The listing builds one solid part. Answer for the finished solid, in the listing's coordinates (mm). Face numbers are marked on the shaded views. A direction names the side the tool comes from. Coordinates: 2 decimals unless noted, no trailing zeros. Order: outer loops, then holes, each group sorted by start corner. A loop starts at its lowest first (then second) coordinate and runs counter-clockwise, first axis right, second up.
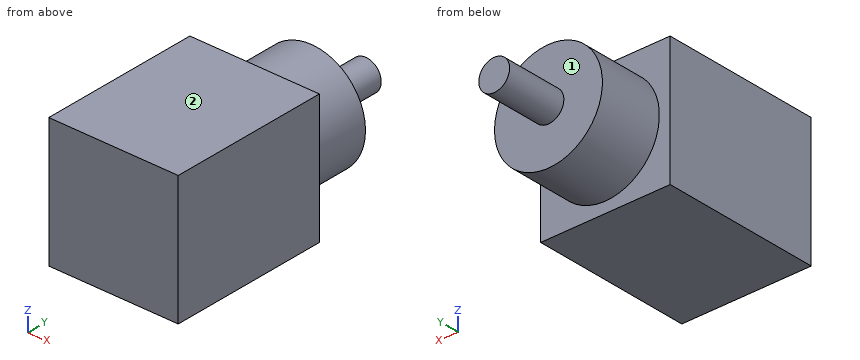
Autodesk Inventor part; units mm, degrees
ref_plane "YZ Plane" through (0, 0, 0) normal (1, 0, 0) x (0, 1, 0)
ref_plane "XZ Plane" through (0, 0, 0) normal (0, 1, 0) x (-1, 0, 0)
ref_plane "XY Plane" through (0, 0, 0) normal (0, 0, 1) x (1, 0, 0)
sketch "Sketch1" plane through (0, 0, 0) normal (0, 1, 0) x (-1, 0, 0)
  line L0 (-21, 21) -> (21, 21)
  line L1 (21, 21) -> (21, -21)
  line L2 (21, -21) -> (-21, -21)
  line L3 (-21, -21) -> (-21, 21)
  line L4 (-21, 21) -> (21, -21) construction
  line L5 (21, 21) -> (-21, -21) construction
  point P0 (0, 0)
  dimension "d0" = 42
  dimension "d1" = 42
extrude "Extrusion1" add sketch "Sketch1" along normal blind 52
sketch "Sketch2" plane through (0, 52, 0) normal (0, 1, 0) x (1, 0, 0)
  circle A0 centre (0, 0) radius 17.5
  circle A1 centre (0, 0) radius 5
  dimension "d4" = 35
  dimension "d7" = 10
extrude "Extrusion2" add sketch "Sketch2" along normal blind 21 contours A0 | A1
sketch "Sketch3" plane through (0, 73, 0) normal (0, 1, 0) x (1, 0, 0)
  circle A0 centre (0, 0) radius 5
  dimension "d8" = 10
extrude "Extrusion3" add sketch "Sketch3" along normal blind 20
properties part number "StepperMotor"
1) Section A-A (x = 0) is taken. Give the vertices of the cut face in (y, z).
2) Each of these flat-tipped pins is pushed along its axis until it touches: P1, Ø1.5, axis at x = 16.5, z = -12, coming from the +Y side; P2, Ø10, axis at y = 55.5, z = 10, coming from the -X side; P3, Ø10, axis at x = -6.5, y = 74.5, coming from the +Z side; P4, Ø1.5, axis at y = 73.5, z = 11.5, coming from the +X side. Where does it stop, or does it pass through?
3) A tool of negligible diameter and unlimited length cuts with its end or side. For the marked faces 1 and 2, from which of +Z, -Z, +X, -X, +Y, -Y can it reach the whole face along a straight path? Write none if from no direction.
4) Section B-B (z = -10.5) is taken. Give the vertices of the cut face in (x, y), then the cut area to 3 significant figures.
5) Consider L1, parallel to Y at x = -1, z = -11.5; L2, parallel to Y at x = 8, z = 17; L3, parallel to X at y = 60.5, z = -12.5. Determine where each line is inside the solid, lowest interval first.
6) Section C-C (y = 62) is taken. Give the vertices of the cut face in (x, z), then the cut area to 3 significant figures.
7) Section D-D (z = 0) is taken. Give the vertices of the cut face in (x, y).
Filled sheet:
1. outline: (0, -21) - (52, -21) - (52, -17.5) - (73, -17.5) - (73, -5) - (93, -5) - (93, 5) - (73, 5) - (73, 17.5) - (52, 17.5) - (52, 21) - (0, 21) - close
2. P1: stops at y = 52
2. P2: stops at x = -21
2. P3: stops at z = 17.41
2. P4: stops at x = 13.66
3. face 1: +Y
3. face 2: +Z, +X, -X, +Y, -Y
4. outline: (-21, 0) - (21, 0) - (21, 52) - (14, 52) - (14, 73) - (-14, 73) - (-14, 52) - (-21, 52) - close
4. area: 2,770 mm2
5. L1: y = 0 to 73
5. L2: y = 0 to 52
5. L3: x = -12.25 to 12.25
6. outline: circle Ø35 at (0, 0)
6. area: 962 mm2
7. outline: (-21, 0) - (21, 0) - (21, 52) - (17.5, 52) - (17.5, 73) - (5, 73) - (5, 93) - (-5, 93) - (-5, 73) - (-17.5, 73) - (-17.5, 52) - (-21, 52) - close
